The listing builds one solid part. Answer for the finished solid, in the listing's coordinates (mm). Face numbers are marked on the shaded views. Give positions to 0.01 mm unless a question says otherwise; leave off trailing zeros. Loops run counter-clockwise (first coordinate to the right, second up) from the corner with the lowest first, then second, coordinate; pieces in that order, holes last. Notation, with made-up numbers: M 50.5,53 L 86.5,53 A35 cw 86.5,90 Z; hole C 68.25,-25.75 d3. An arc over 180 degrees is marked long. One line per item, written item: value. Start each with the question number.
Q1. A cutting plane is placed at A-A, the plane z = 0. Determine the outline of the cut face in (x, y), and give its area (3 significant figures).
Q2. Consider L1, parallel to X at y = 2.4, z = 0; L2, parallel to Z at x = 6.5, y = 2.05; L3, parallel to X at y = 3.8, z = -5.5. Determine where each line is inside the solid, lowest interval first.
Q3. A flat-ended cylindrical pin translates along its axis: pin 1 (2 mm diameter, centred on y = 2.5, z = -5.5, fed in from -X). Find the tip coordinate at first contact, or state that the pin passes through.
Q4. The mould has two halves that part along X. Classify the marked faces 1, 2 and 3: +X half, -X half, draft (parallel to the pull), parting line (faces both ways), or undercut.
Q5. A cutting plane is placed at B-B, the plane x = 2. Determine the outline of the cut face in (y, z).
Q6. A cutting plane is placed at C-C, the plane y = 3.75. Determine the outline of the cut face in (x, z), and give its area (3 significant figures).
from build123d import *

# Parameters (mm, degrees)
SALIENTE_EXTRUIR1_DEPTH = 5
CROQUIS2_R              = 7.8
CORTAR_EXTRUIR1_DEPTH   = 5


with BuildPart() as part:
    # Croquis1 → Saliente-Extruir1 (new body)
    with BuildSketch(Plane(origin=(0, 0, 0), x_dir=(1, 0, 0), z_dir=(0, 1, 0))):
        with BuildLine():
            Line((0, -10), (30, -10))
            Line((30, -10), (30, 10))
            Line((30, 10), (0, 10))
            ThreePointArc((0, 10), (-10, 0), (0, -10))
        make_face()
    extrude(amount=SALIENTE_EXTRUIR1_DEPTH)

    # Croquis2 → Cortar-Extruir1 (cut)
    with BuildSketch(Plane(origin=(0, 5, 0), x_dir=(1, 0, 0), z_dir=(0, 1, 0))):
        with Locations(Location((0, 0, 0), (0, 0, 270))):
            Circle(CROQUIS2_R)
    extrude(amount=-CORTAR_EXTRUIR1_DEPTH, mode=Mode.SUBTRACT)


solid = part.part
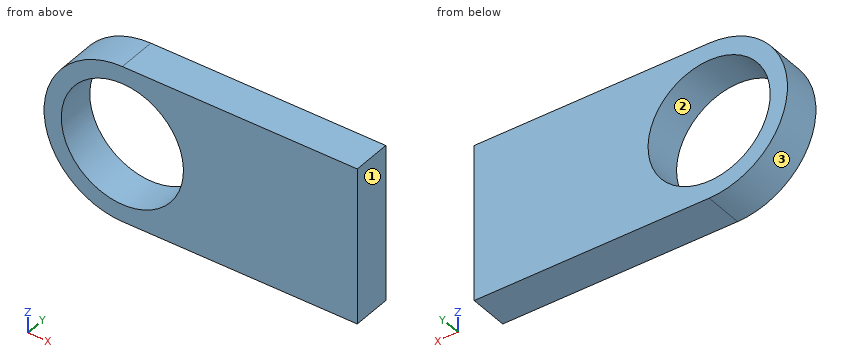
Answer block:
1. outline: M -10,0 L -7.8,0 L -7.8,5 L -10,5 Z; M 7.8,0 L 30,0 L 30,5 L 7.8,5 Z
1. area: 122 mm^2
2. L1: -10 to -7.8, 7.8 to 30
2. L2: -10 to -4.31, 4.31 to 10
2. L3: -8.35 to -5.53, 5.53 to 30
3. pin 1: x = -8.93
4. face 1: +X half
4. face 2: undercut
4. face 3: -X half
5. outline: M 0,-10 L 5,-10 L 5,-7.54 L 0,-7.54 Z; M 0,7.54 L 5,7.54 L 5,10 L 0,10 Z
6. outline: M 0,-10 L 30,-10 L 30,10 L 0,10 A10 ccw Z; hole C 0,0 d15.6
6. area: 566 mm^2
